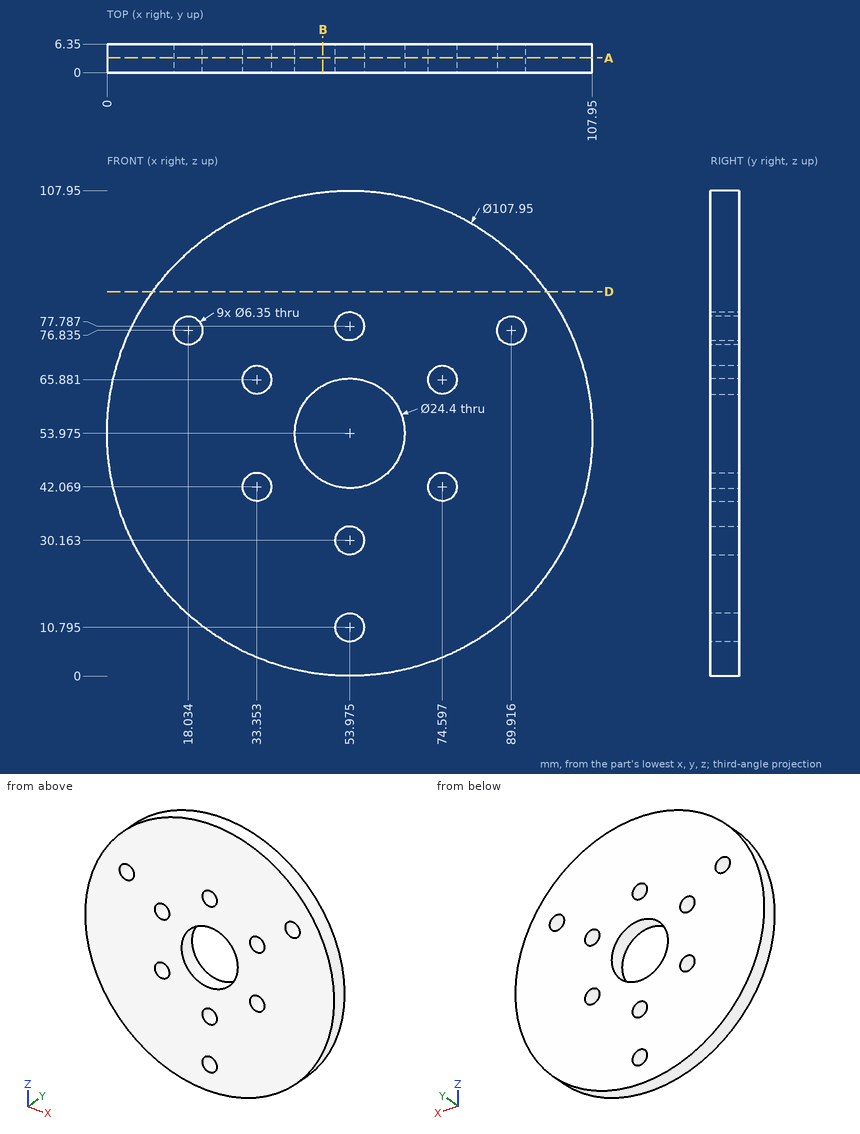
Job drawing, mm, ordinate dimensions from the low corner. One solid piece. Give positions to 0.01 mm unless a question says otherwise; leave off trailing zeros. Loops run counter-clockwise (first coordinate to the right, second up) from the corner with the lowest first, then second, coordinate; pieces in that order, holes last.
Item 1: Slice it at D-D, the plane z = 85.5. List the corners of the cut face in (x, y).
Answers follow:
outline: (10.16, 0) - (97.79, 0) - (97.79, 6.35) - (10.16, 6.35) - close
Item 2: Slice it at A-A, the plane y = 3.25. Give the number of separate pieces and of enclosed holes in the cut face, and give its area (3 significant figures).
Answers follow:
separate pieces: 1
enclosed holes: 10
area: 8,400 mm2
Item 3: Slice it at B-B, the plane x = 48. List the corners of the cut face in (y, z), and give its area (3 significant figures).
Answers follow:
outline: (0, 0.33) - (6.35, 0.33) - (6.35, 43.34) - (0, 43.34) - close; (0, 64.61) - (6.35, 64.61) - (6.35, 107.62) - (0, 107.62) - close
area: 546 mm2
Item 4: Flat gauge pins, fed straight in: pin 1 (1 mm diameter, centred on x = 87.5, y = 1, fed in from -Z); pin 2 (3 mm diameter, centred on y = 1, z = 88, fed in from -X). Where does each tip first touch, or does it go through?
Answers follow:
pin 1: stops at z = 11.28
pin 2: stops at x = 10.9
Item 5: Drill centre lines: line 1 (Z direction, x = 33, y = 1) (1 decimal); line 2 (X direction, y = 0.5, z = 80.5) (1 decimal); line 3 (Z direction, x = 64, y = 6) (1 decimal). Where is each one in solid material? Low to high.
Answers follow:
line 1: z = 4.2 to 38.9, 45.2 to 62.7, 69 to 103.7
line 2: x = 7 to 52.3, 55.6 to 101
line 3: z = 0.9 to 47, 60.9 to 107
